Input: dimensioned drawing with shaded views. Units: mm. Origin: part minimum x, y, z. Coordinates: 2 decimals unless noted, no trailing zeros. Loops run counter-clockwise (first coordinate to the right, second up) from the corner with the lowest first, then second, coordinate; pieces in that order, holes last. Notation, with made-up numbers: (72, 21.25) -> (125, 21.25) arc R16 cw to (125, 25.25) -> close; hole circle Ø5 at (-12.75, 81.25). An arc over 180 degrees is marked (long way). Answer as CSV lines item,"result".
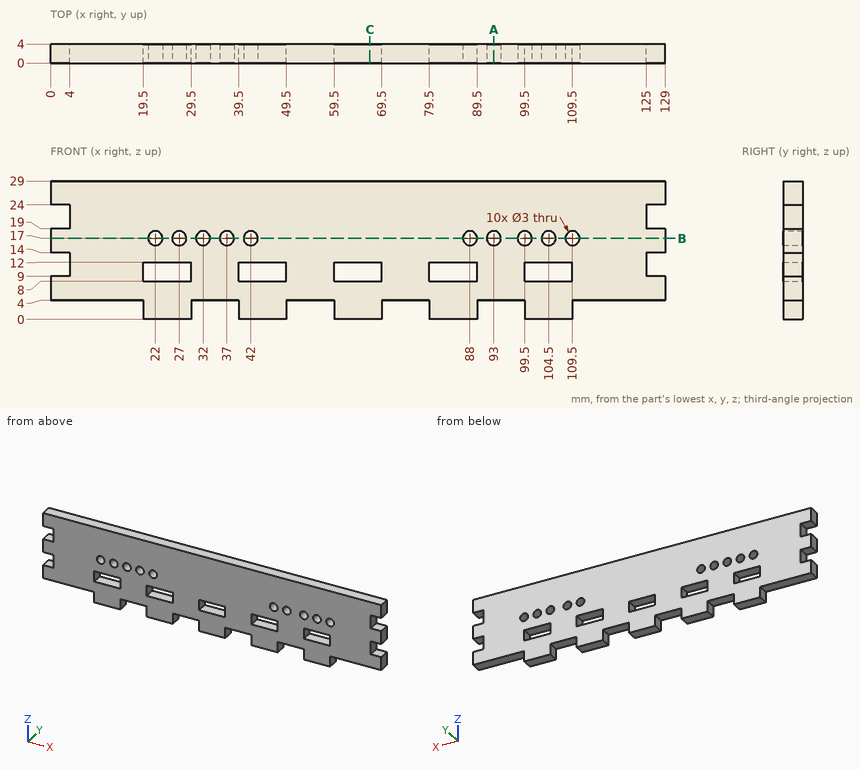
(1) Cut plane B-B (z = 17). State how many separate pieces and enclosed holes the cut face has, then the cut area to 3 significant figures.
Computed values:
separate pieces,"11"
enclosed holes,"0"
area,"396 mm^2"
(2) Cut plane C-C (x = 67). Return the cut outline in (y, z), then the cut area to 3 significant figures.
Computed values:
outline,"(0, 0) -> (4, 0) -> (4, 8) -> (0, 8) -> close; (0, 12) -> (4, 12) -> (4, 29) -> (0, 29) -> close"
area,"100 mm^2"
(3) Material intervals for L1, parallel to X at y = 2.9, z = 2.25; L2, parallel to Z at x = 44.5, y = 0.5; L3, parallel to X at y = 1.4, z = 9.25, sorted ascending. Write a range as [from, to].
Computed values:
L1,"[19.5, 29.5], [39.5, 49.5], [59.5, 69.5], [79.5, 89.5], [99.5, 109.5]"
L2,"[0, 8], [12, 29]"
L3,"[4, 19.5], [29.5, 39.5], [49.5, 59.5], [69.5, 79.5], [89.5, 99.5], [109.5, 125]"
(4) Cut plane A-A (x = 93). Return the cut outline in (y, z).
Computed values:
outline,"(0, 4) -> (4, 4) -> (4, 15.5) -> (0, 15.5) -> close; (0, 18.5) -> (4, 18.5) -> (4, 29) -> (0, 29) -> close"
(5) Pin query (flat end, axial travel): pin 1 Ø2 at (x, y) = (3, 1) entering from -Z; pin 2 Ø2 at (y, z) = (2.5, 11) entering from +X; pin 3 Ø1.2 at (y, z) = (1.5, 1.5) entering from +X. Return the tip coordinate at first contact, or that it passes through.
Computed values:
pin 1,"z = 4"
pin 2,"x = 125"
pin 3,"x = 109.5"
